Work out the finished part from the listing and answer in its coordinate system (mm). A direction names the side the tool comes from. Coordinates: 2 decimals unless noted, no trailing zeros. Loops run counter-clockwise (first coordinate to the right, second up) from the corner with the lowest first, then second, coordinate; pieces in that order, holes last.
```python
from build123d import *

# Parameters (mm, degrees)
SKETCH1_R           = 70
BOSS_EXTRUDE1_DEPTH = 7
SKETCH2_R           = 55
SKETCH2_R_2         = 50
BOSS_EXTRUDE2_DEPTH = 3
SKETCH3_R           = 3
CUT_EXTRUDE1_DEPTH  = 11


with BuildPart() as part:
    # Sketch1 → Boss-Extrude1 (new body)
    with BuildSketch(Plane.XY):
        Circle(SKETCH1_R)
    extrude(amount=BOSS_EXTRUDE1_DEPTH)

    # Sketch2 → Boss-Extrude2 (add)
    with BuildSketch(Plane(origin=(0, 0, 0), x_dir=(-1, 0, 0), z_dir=(0, 0, -1))):
        Circle(SKETCH2_R)
        Circle(SKETCH2_R_2, mode=Mode.SUBTRACT)
    extrude(amount=BOSS_EXTRUDE2_DEPTH)

    # Sketch3 → Cut-Extrude1 (cut, through all)
    with BuildSketch(Plane.XY.offset(7)):
        with Locations((0, 60)):
            Circle(SKETCH3_R)
        with Locations((51.961524227, -30)):
            Circle(SKETCH3_R)
        with Locations((-51.961524227, -30)):
            Circle(SKETCH3_R)
    extrude(amount=-CUT_EXTRUDE1_DEPTH, mode=Mode.SUBTRACT)


solid = part.part
```
1. A cutting plane is placed at C-C, the plane z = 2.25. Give the vertices of the cut face in (x, y), then the cut area to 3 significant figures.
2. Each of these flat-tipped pins is pushed along its axis until it touches: P1, Ø4, axis at x = 25, z = 1, coming from the +Y side; P2, Ø1.5, axis at x = -53, y = -22.5, coming from the -Z side; P3, Ø6, axis at x = 4, z = 5, coming from the -Y side. Where does it stop, or does it pass through?
3. For faces 1 (the flat face through (-1, 1, 0)), 2 (the cylindrical face through (0, 63, 4)), determine the directions among +Z, -Z, +X, -X, +Y, -Y from which every point of the face is accessible in a straight line to the end or side of a thin tool.
4. A cutting plane is placed at B-B, the plane y = -30. Give the vertices of the cut face in (x, z), then the cut area to 3 significant figures.
5. A cutting plane is placed at A-A, the plane x = 0. Give the vertices of the cut face in (y, z), then the cut area to 3 significant figures.
6. A cutting plane is placed at D-D, the plane y = 60. Give the vertices of the cut face in (x, z).
7. Determine the mould class of faces 3 (the cylindrical face through (11.923, -53.692, -1.479)), 4 (the cylindrical face through (-47.69, 15.02, -1.48)), 5 (the flat face through (36, 42, 0)) for opening direction X: released by +X, released by -X, zero draft, split by the parting line, or undercut.
8. Straight lines are drawn through the part: probe 1 along Y at (x, z) = (0, -1.6); probe 2 along Z at (x, y) = (-62, 30); probe 3 along Y at (x, z) = (13.5, -0.25). For each, find the intervals that lie inside material, in ascending order.
Answers below:
1. outline: circle Ø140 at (0, 0); hole circle Ø6 at (-51.96, -30); hole circle Ø6 at (0, 60); hole circle Ø6 at (51.96, -30)
1. area: 15,300 mm2
2. P1: stops at y = 66.11
2. P2: stops at z = 0
2. P3: stops at y = -69.99
3. face 1: -Z
3. face 2: +Z, -Z
4. outline: (-63.25, 0) - (-54.96, 0) - (-54.96, 7) - (-63.25, 7) - close; (-48.96, 0) - (-46.1, 0) - (-46.1, -3) - (-40, -3) - (-40, 0) - (40, 0) - (40, -3) - (46.1, -3) - (46.1, 0) - (48.96, 0) - (48.96, 7) - (-48.96, 7) - close; (54.96, 0) - (63.25, 0) - (63.25, 7) - (54.96, 7) - close
4. area: 838 mm2
5. outline: (-70, 0) - (-55, 0) - (-55, -3) - (-50, -3) - (-50, 0) - (50, 0) - (50, -3) - (55, -3) - (55, 0) - (57, 0) - (57, 7) - (-70, 7) - close; (63, 0) - (70, 0) - (70, 7) - (63, 7) - close
5. area: 968 mm2
6. outline: (-36.06, 0) - (-3, 0) - (-3, 7) - (-36.06, 7) - close; (3, 0) - (36.06, 0) - (36.06, 7) - (3, 7) - close
7. face 3: split by the parting line
7. face 4: undercut
7. face 5: zero draft
8. probe 1: y = -55 to -50, 50 to 55
8. probe 2: z = 0 to 7
8. probe 3: y = -53.32 to -48.14, 48.14 to 53.32
